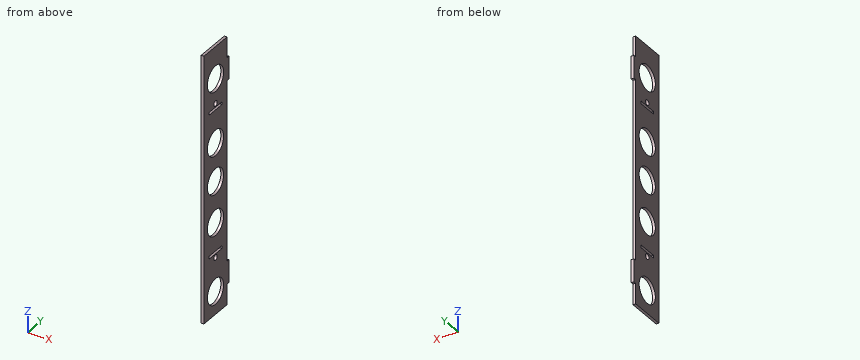
```python
from build123d import *

# Parameters (mm, degrees)
SKETCH3_W           = 292
SKETCH3_H           = 40
SKETCH3_W_2         = 3
SKETCH3_H_2         = 22
SKETCH3_W_3         = 25
SKETCH3_H_3         = 3
BOSS_EXTRUDE2_DEPTH = 3
SKETCH5_R           = 14
CUT_EXTRUDE1_DEPTH  = 10
SKETCH6_R           = 3
CUT_EXTRUDE2_DEPTH  = 10


with BuildPart() as part:
    # Sketch3 → Boss-Extrude2 (new body)
    with BuildSketch(Plane(origin=(0, 0, 0), x_dir=(0, 0, -1), z_dir=(1, 0, 0))):
        with Locations((146, -20)):
            Rectangle(SKETCH3_W, SKETCH3_H)
        with Locations((67.54, -20)):
            Rectangle(SKETCH3_W_2, SKETCH3_H_2, mode=Mode.SUBTRACT)
        with Locations((224.46, -20)):
            Rectangle(SKETCH3_W_2, SKETCH3_H_2, mode=Mode.SUBTRACT)
        with Locations((35, 1.5)):
            Rectangle(SKETCH3_W_3, SKETCH3_H_3)
        with Locations((257, 1.5)):
            Rectangle(SKETCH3_W_3, SKETCH3_H_3)
    extrude(amount=BOSS_EXTRUDE2_DEPTH)

    # Sketch5 → Cut-Extrude1 (cut)
    with BuildSketch(Plane(origin=(3, 0, 0), x_dir=(0, 0, -1), z_dir=(1, 0, 0))):
        with Locations((35, -20)):
            Circle(SKETCH5_R)
        with Locations((105, -20)):
            Circle(SKETCH5_R)
        with Locations((147, -20)):
            Circle(SKETCH5_R)
        with Locations((192, -20)):
            Circle(SKETCH5_R)
        with Locations((267, -20)):
            Circle(SKETCH5_R)
    extrude(amount=-CUT_EXTRUDE1_DEPTH, mode=Mode.SUBTRACT)

    # Sketch6 → Cut-Extrude2 (cut)
    with BuildSketch(Plane(origin=(3, 0, 0), x_dir=(0, 0, -1), z_dir=(1, 0, 0))):
        with Locations((62, -20)):
            Circle(SKETCH6_R)
        with Locations((230, -20)):
            Circle(SKETCH6_R)
    extrude(amount=-CUT_EXTRUDE2_DEPTH, mode=Mode.SUBTRACT)


solid = part.part
```
Work out the finished part from the listing and answer in its coordinate system (mm). Give positions to 0.01 mm unless a question says otherwise; leave off trailing zeros. Write each loop counter-clockwise with the first axis right and the second up, starting at its lowest first coordinate (ties: lowest second). Pieces come first, ordered by that corner, then holes. Notation, with made-up numbers: (24.5, 53.25) - (69.5, 53.25) arc R22 cw to (69.5, 83.25) - close; hole circle Ø10 at (32, 64). An arc over 180 degrees is marked (long way). Use one line per item in the form item = value.
1. Each of these flat-tipped pins is pushed along its axis until it touches: pin 1 Ø0.9 at (x, z) = (1.5, -158.5) entering from +Y; pin 2 Ø0.9 at (x, y) = (1.5, 2) entering from -Z. Where does it stop, or does it pass through?
Filled in:
pin_1 = 0
pin_2 = -269.5
2. A cutting plane is placed at B-B (x = 1.75). State how many separate pieces and enclosed holes the cut face has, and give its area (3 significant figures).
Filled in:
separate_pieces = 1
enclosed_holes = 9
area = 8,560 mm^2
3. A cutting plane is placed at D-D (z = -62). Write down the section's boundary in (x, y), and give its area (3 significant figures).
Filled in:
outline = (0, -40) - (3, -40) - (3, -23) - (0, -23) - close; (0, -17) - (3, -17) - (3, 0) - (0, 0) - close
area = 102 mm^2
4. A cutting plane is placed at A-A (z = -192). Write down the section's boundary in (x, y), and give its area (3 significant figures).
Filled in:
outline = (0, -40) - (3, -40) - (3, -34) - (0, -34) - close; (0, -6) - (3, -6) - (3, 0) - (0, 0) - close
area = 36.0 mm^2
5. Consider L1, parallel to Y at x = 1.3, z = -105; L2, parallel to Y at x = 1.15, z = -230; L3, parallel to Y at x = 1.35, z = -177. Determine where each line is inside the solid, lowest interval first.
Filled in:
L1 = -40 to -34, -6 to 0
L2 = -40 to -23, -17 to 0
L3 = -40 to 0
